from build123d import *

# Parameters (mm, degrees)
EXTRUDE1_DEPTH         = 12
M10_GEVINDHULLER_D     = 8.5
M10_GEVINDHULLER_DEPTH = 22
M10_GEVINDHULLER_TIP   = 2.553657631


with BuildPart() as part:
    # Sketch1 → Extrude1 (new body)
    with BuildSketch(Plane.XY):
        with BuildLine():
            Line((36.5, 6.420773039), (36.5, 3))
            ThreePointArc((36.5, 3), (35.621320344, 0.878679656), (33.5, 0))
            Line((33.5, 0), (0, 0))
            Line((0, 0), (-33.5, 0))
            ThreePointArc((-33.5, 0), (-35.621320344, 0.878679656), (-36.5, 3))
            Line((-36.5, 3), (-36.5, 6.420773039))
            ThreePointArc((-36.5, 6.420773039), (-37.624306556, 11.49219218), (-40.786548684, 15.613306357))
            Line((-40.786548684, 15.613306357), (-72.713451316, 42.40315858))
            ThreePointArc((-72.713451316, 42.40315858), (-75.875693444, 46.524272757), (-77, 51.595691898))
            Line((-77, 51.595691898), (-77, 73))
            ThreePointArc((-77, 73), (-75.611898825, 75.530174337), (-72.732145215, 75.718923361))
            Line((-72.732145215, 75.718923361), (-8.939617358, 45.971979088))
            ThreePointArc((-8.939617358, 45.971979088), (-8.345295598, 45.605139594), (-7.851901649, 45.110819879))
            ThreePointArc((-7.851901649, 45.110819879), (0, 41.303367053), (7.851901649, 45.110819879))
            ThreePointArc((7.851901649, 45.110819879), (8.345295598, 45.605139594), (8.939617358, 45.971979088))
            Line((8.939617358, 45.971979088), (72.732145215, 75.718923361))
            ThreePointArc((72.732145215, 75.718923361), (75.611898825, 75.530174337), (77, 73))
            Line((77, 73), (77, 51.595691898))
            ThreePointArc((77, 51.595691898), (75.875693444, 46.524272757), (72.713451316, 42.40315858))
            Line((72.713451316, 42.40315858), (40.786548684, 15.613306357))
            ThreePointArc((40.786548684, 15.613306357), (37.624306556, 11.49219218), (36.5, 6.420773039))
        make_face()
    extrude(amount=EXTRUDE1_DEPTH)

    # M10 gevindhuller
    with Locations(Plane.XY.offset(12)):
        with Locations((-33, 43.950984745), (-56.564002463, 54.93905955), (56.564002463, 54.93905955), (33, 43.950984745)):
            Hole(M10_GEVINDHULLER_D / 2, depth=M10_GEVINDHULLER_DEPTH)
            with Locations((0, 0, -(M10_GEVINDHULLER_DEPTH + M10_GEVINDHULLER_TIP / 2))):  # 118° drill point
                Cone(0, M10_GEVINDHULLER_D / 2, M10_GEVINDHULLER_TIP, mode=Mode.SUBTRACT)


solid = part.part
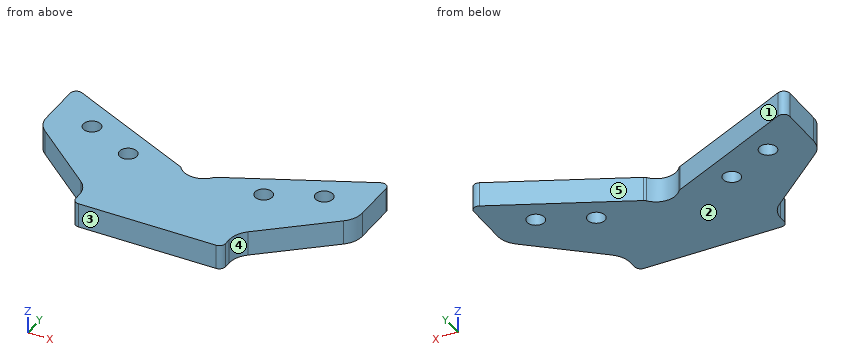
Input: part model. Units: mm. Frame: model coordinates. Face numbers are marked on the shaded views. A direction names the side the tool comes from. Coordinates: 2 decimals unless noted, no trailing zeros. Loops run counter-clockwise (first coordinate to the right, second up) from the corner with the lowest first, then second, coordinate; pieces in that order, holes last. Notation, with made-up numbers: (-26.5, 47) -> (16.5, 47) arc R30 cw to (16.5, 74) -> close; hole circle Ø8 at (35.25, 67). An arc over 180 degrees is marked (long way). Write item = value, one per line. Start each with the question number.
Item 1: Reachability of the marked faces 1 and 2 from +Z, -Z, +X, -X, +Y, -Y: full face, straight path, thin tool, end or side. Return the list, or none.
Item 2: Cut plane C-C, the plane z = 4.25. Return loops of the section in (x, y).
Item 3: Cut plane B-B, the plane x = -35. Return loops of the section in (y, z), plus the area to 3 significant figures.
Item 4: Mould query, pull axis X, two halves, no side actions, for the marked faces 3, 4 and 5. Classes: pulls with the +X half, pulls with the -X half, needs draft (parallel to the pull), parting line crosses it, or undercut.
Item 5: Material intervals for line 1 (X direction, y = 56, z = 1.5); line 2 (X direction, y = 54, z = 0.5); line 3 (X direction, y = 4, z = 6.75), sorted ascending.
Item 6: Cut plane A-A, the plane y = 63.5. Return loops of the section in (x, z), plus the area to 3 significant figures.
Item 7: Cut plane D-D, the plane x = 23.5. Return loops of the section in (y, z).
Item 8: First-contact query: P1, Ø7, axis at x = 56.56, y = 54.94, coming from the +Z side; P2, Ø1.7, axis at y = 5.5, z = 8, coming from the -X side; P3, Ø2, axis at y = 18, z = 2.5, coming from the +X side; P4, Ø3, axis at y = 17.5, z = 6.5, coming from the -X side. Flat tips, straight axial feed; report the tip coordinate or a pass-through.
Ans:
q1.face_1 = +Z, -Z, +Y
q1.face_2 = -Z, +X, -X, +Y, -Y
q2.outline = (-77, 51.6) arc R12 ccw to (-72.71, 42.4) -> (-40.79, 15.61) arc R12 cw to (-36.5, 6.42) -> (-36.5, 3) arc R3 ccw to (-33.5, 0) -> (33.5, 0) arc R3 ccw to (36.5, 3) -> (36.5, 6.42) arc R12 cw to (40.79, 15.61) -> (72.71, 42.4) arc R12 ccw to (77, 51.6) -> (77, 73) arc R3 ccw to (72.73, 75.72) -> (8.94, 45.97) arc R3 ccw to (7.85, 45.11) arc R10 cw to (-7.85, 45.11) arc R3 ccw to (-8.94, 45.97) -> (-72.73, 75.72) arc R3 ccw to (-77, 73) -> close; hole circle Ø8.5 at (-56.56, 54.94); hole circle Ø8.5 at (-33, 43.95); hole circle Ø8.5 at (33, 43.95); hole circle Ø8.5 at (56.56, 54.94)
q3.outline = (0.4, 0) -> (40.2, 0) -> (40.2, 12) -> (0.4, 12) -> close; (47.7, 0) -> (58.12, 0) -> (58.12, 12) -> (47.7, 12) -> close
q3.area = 603 mm²
q4.face_3 = needs draft
q4.face_4 = pulls with the +X half
q4.face_5 = undercut
q5.line_1 = -77 to -60.68, -52.45 to -30.44, 30.44 to 52.45, 60.68 to 77
q5.line_2 = -77 to -60.71, -52.42 to -26.16, 26.16 to 52.42, 60.71 to 77
q5.line_3 = -36.5 to 36.5
q6.outline = (-77, 0) -> (-46.53, 0) -> (-46.53, 12) -> (-77, 12) -> close; (46.53, 0) -> (77, 0) -> (77, 12) -> (46.53, 12) -> close
q6.area = 731 mm²
q7.outline = (0, 0) -> (52.76, 0) -> (52.76, 12) -> (0, 12) -> close
q8.P1 = through
q8.P2 = -36.5
q8.P3 = 44.82
q8.P4 = -44.82
